Check sheet for the drawn part. Datum: minimum x, y, z corner. Units: mm. A direction names the side the tool comes from. Round coordinates to 2 decimals unless told otherwise and drop trailing zeros. Order: outer loops, then holes, each group sorted by start corner. A loop starts at its lowest first (then second) coordinate and runs counter-clockwise, first axis right, second up. Notation, with made-up numbers: (89, -29.5) - (118, -29.5) arc R26 ccw to (118, -12.5) - close; hole circle Ø10 at (-26.75, 59). An arc over 180 degrees is marked (long way). Write each question's results on one line, items separated by ' | '.
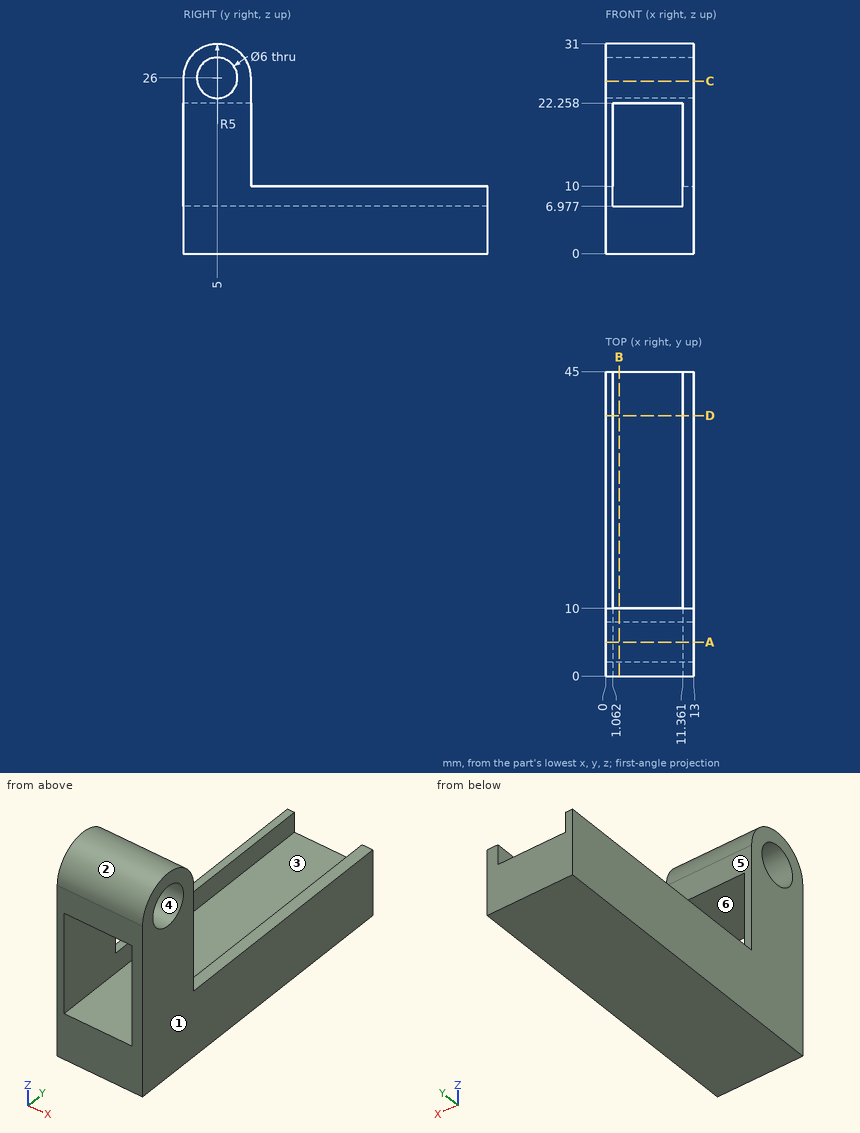
(1) Section check B-B (x = 2). Record the cut outline in (y, z), then the cut area to 3 significant figures.
Answers follow:
outline: (0, 0) - (45, 0) - (45, 6.98) - (0, 6.98) - close; (0, 22.26) - (10, 22.26) - (10, 26) arc R5 ccw to (0, 26) - close; hole circle Ø6 at (5, 26) | area: 362 mm²
(2) Material ranges on line 1 (Z direction, x = 6, y = 5); line 2 (X direction, y = 8.5, z = 20); line 3 (Z direction, x = 1.5, y = 35.5), recorded low to high.
Answers follow:
line 1: 0 to 6.98, 22.26 to 23, 29 to 31 | line 2: 0 to 1.06, 11.36 to 13 | line 3: 0 to 6.98
(3) Depth check by flat-ended pin: pin 1 Ø3 at (x, y) = (5, 13.5) entering from +Z; pin 2 Ø6.5 at (x, z) = (9.5, 17) entering from +Y; pin 3 Ø5 at (y, z) = (5, 26) entering from -X; pin 4 Ø0.8 at (x, y) = (0.5, 20) entering from +Z. Enter the tip coordinate at first touch or a pass-through.
Answers follow:
pin 1: z = 6.98 | pin 2: y = 10 | pin 3: through | pin 4: z = 10
(4) Section check C-C (z = 25.5). Record the cut outline in (x, y), then the cut area to 3 significant figures.
Answers follow:
outline: (0, 0) - (13, 0) - (13, 2.04) - (0, 2.04) - close; (0, 7.96) - (13, 7.96) - (13, 10) - (0, 10) - close | area: 53.1 mm²
(5) Section check D-D (y = 38.5). Record the cut outline in (x, z).
Answers follow:
outline: (0, 0) - (13, 0) - (13, 10) - (11.36, 10) - (11.36, 6.98) - (1.06, 6.98) - (1.06, 10) - (0, 10) - close
(6) Draft check along Z on the marked faces 1, 2 and 3. Enter one of: released by +Z, released by -Z, zero draft, split by the parting line, or undercut.
Answers follow:
face 1: zero draft | face 2: released by +Z | face 3: undercut
(7) Access from +Z, -Z, +X, -X, +Y, -Y to the whole of each face (thin tool, end or side, straight path). Record for the marked faces 4, 5 and 6.
Answers follow:
face 4: +X, -X | face 5: +Z, +X, -X, +Y | face 6: +Y, -Y
(8) Section check A-A (y = 5). Record the cut outline in (x, z), then the cut area to 3 significant figures.
Answers follow:
outline: (0, 0) - (13, 0) - (13, 23) - (0, 23) - close; (0, 29) - (13, 29) - (13, 31) - (0, 31) - close; hole (1.06, 6.98) - (11.36, 6.98) - (11.36, 22.26) - (1.06, 22.26) - close | area: 168 mm²
